Verification items for the finished model (mm, model axes). Face numbers are marked on the shaded views. Coordinates: 2 decimals unless noted, no trailing zeros. Write each loop counter-clockwise with the first axis right and the second up, starting at its lowest first coordinate (ties: lowest second). Pieces come first, ordered by that corner, then holes. Notation, with made-up numbers: (67.25, 42.5) - (108.25, 42.5) arc R12 cw to (108.25, 47.5) - close; hole circle Ø2 at (40.5, 73.25). An arc over 180 degrees is marked (long way). Use CSV: the item, a comma, the result in double quotes. Start each with the question number.
```python
from build123d import *

# Parameters (mm, degrees)
BOSS_EXTRUDE1_DEPTH     = 7
SKETCH3_W               = 15
SKETCH3_H               = 7
BOSS_EXTRUDE2_DEPTH     = 3.5
CUT_EXTRUDE1_DEPTH      = 1
CUT_EXTRUDE1_DEPTH_BACK = 16
FILLET1_R               = 2


with BuildPart() as part:
    # Sketch1 → Boss-Extrude1 (new body)
    with BuildSketch(Plane.XY):
        Polygon((-7.5, -6), (7.5, 6), (-7.5, 6), align=None)
    extrude(amount=BOSS_EXTRUDE1_DEPTH)

    # Sketch3 → Boss-Extrude2 (add)
    with BuildSketch(Plane(origin=(0, 6, 0), x_dir=(1, 0, 0), z_dir=(0, 1, 0))):
        with Locations((0, -3.5)):
            Rectangle(SKETCH3_W, SKETCH3_H)
    extrude(amount=BOSS_EXTRUDE2_DEPTH)

    # Sketch4 → Cut-Extrude1 (cut, two sides)
    with BuildSketch(Plane(origin=(7.5, 0, 0), x_dir=(0, 0, -1), z_dir=(1, 0, 0))) as cut_extrude1_sk:
        with BuildLine():
            Line((-6.5, 53.115472628), (-6.5, 9.5))
            ThreePointArc((-6.5, 9.5), (-3.5, 6.5), (-0.5, 9.5))
            Line((-0.5, 9.5), (-0.5, 53.115472628))
            Line((-0.5, 53.115472628), (-0.5, 140.346417884))
            Line((-0.5, 140.346417884), (-6.5, 140.346417884))
            Line((-6.5, 140.346417884), (-6.5, 53.115472628))
        make_face()
    extrude(amount=CUT_EXTRUDE1_DEPTH, mode=Mode.SUBTRACT)
    extrude(cut_extrude1_sk.sketch, amount=-CUT_EXTRUDE1_DEPTH_BACK, mode=Mode.SUBTRACT)

    # Fillet1
    fillet1_edges = [part.edges().sort_by_distance(p)[0] for p in [
        (0, 0, 0),
        (0, 0, 7),
    ]]
    fillet(fillet1_edges, radius=FILLET1_R)


solid = part.part
```
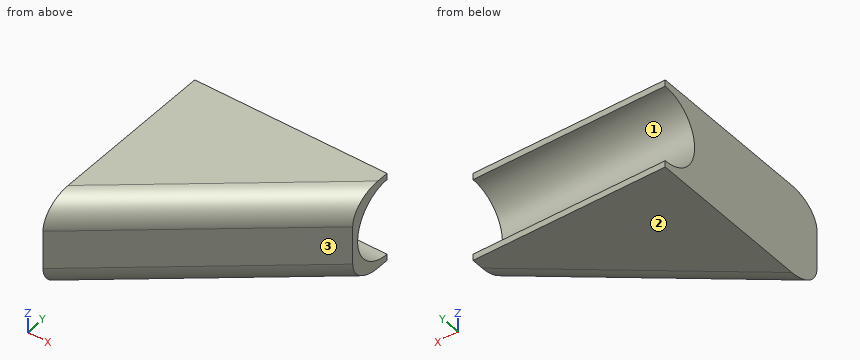
Q1. Cross-section at A-A (z = 3.5). Record the cut outline in (x, y), plus the area to 3 significant figures.
Q2. Cross-section at B-B (z = 1). Record the cut outline in (x, y).
Q3. Gauge pin test, flat ends, axial feed: pin 1 (3 mm diameter, centred on x = 0, z = 4.5, fed in from -Y); pin 2 (2 mm diameter, centred on x = -4, z = 4.5, fed in from -Y); pin 3 (2 mm diameter, centred on y = 3, z = 4, fed in from +X). Record the tip position at first contact, or that the pin passes through.
Q4. Scan lines: line 1 along Z through (x, y) = (-6.25, 7); line 2 along Y through (x, z) = (0, 3.5); line 3 along X through (y, z) = (5.75, 4). Record each from-to range of solid material in increasing order. Write a range as from..to.
Q5. Release check for a two-part mould opening along Z. For the marked faces 1, 2 and 3 record: released by +Z, released by -Z, zero draft, split by the parting line, or undercut.
Reply:
1,outline,"(-7.5, -6) - (7.5, 6) - (7.5, 6.5) - (-7.5, 6.5) - close"
1,area,"97.5 mm^2"
2,outline,"(-7.5, -5.66) - (7.5, 6.34) - (7.5, 7.84) - (-7.5, 7.84) - close"
3,pin 1,"y = -1.2"
3,pin 2,"y = -4"
3,pin 3,"x = 5"
4,line 1,"0..1.84, 5.16..7"
4,line 2,"0..6.5"
4,line 3,"-7.5..7.19"
5,face 1,"undercut"
5,face 2,"released by -Z"
5,face 3,"zero draft"
